Autodesk Fusion 360 part; units mm, degrees
sketch "Sketch3" plane through (0, 0, 0) normal (0, 0, 1) x (1, 0, 0)
  circle A0 centre (0, 0) radius 5.75
  dimension "d17" = 11.5
ref_plane "WorkPlane1" through (0, 0, 46) normal (0, 0, 1) x (1, 0, 0)
sketch "Sketch4" plane through (0, 0, 46) normal (0, 0, 1) x (1, 0, 0)
  line L0 (4, -6) -> (-4, -6)
  line L1 (-6, -4) -> (-6, 4)
  line L2 (-4, 6) -> (4, 6)
  line L3 (6, 4) -> (6, -4)
  arc A0 (-4, 6) -> (-6, 4) centre (-4, 4) ccw
  arc A1 (6, 4) -> (4, 6) centre (4, 4) ccw
  arc A2 (4, -6) -> (6, -4) centre (4, -4) ccw
  arc A3 (-6, -4) -> (-4, -6) centre (-4, -4) ccw
  point P0 (-6, -6)
  point P1 (-6, 6)
  point P2 (6, 6)
  dimension "d19" = 12
  dimension "d20" = 12
  dimension "d21" = 6
  dimension "d22" = 6
  dimension "d23" = 2
  dimension "d24" = 2
  dimension "d25" = 2
  dimension "d26" = 2
loft "Loft1" add profiles "Sketch3", "Sketch4" section 1 section 2
sketch "Sketch5" plane through (0, 0, 0) normal (0, 0, -1) x (1, 0, 0)
  circle A0 centre (0, 0) radius 4.75
  arc A1 (4.8644, 3.066) -> (4.8549, -3.081) centre (0, 0) ccw
  arc A2 (4.8549, -3.081) -> (4.8644, 3.066) centre (0, 0) ccw
  dimension "d27" = 9.5
extrude "Extrude2" cut sketch "Sketch5" against normal blind 43 contours A0
fillet "Fillet1" radius 1 2 edges at (6, 0, 46) (-6, 0, 46)
fillet "Fillet2" radius 0.5 1 edges at (-4.4286, -1.7177, 0)
sketch "Sketch1" plane through (0, 0, 0) normal (0, 1, 0) x (1, 0, 0)
  circle A0 centre (0, 0) radius 4.5
  circle A1 centre (0, 0) radius 5.5
  dimension "d1" = 9
  dimension "d2" = 11
extrude "Extrude1" [suppressed]
sketch "Sketch2" plane through (0, 0, 0) normal (0, 0, 1) x (1, 0, 0)
  line L0 (4.75, 0) -> (4.75, 43)
  line L1 (4.75, 43) -> (0, 43)
  line L2 (0, 43) -> (0, 45)
  line L3 (0, 45) -> (5.75, 45)
  line L4 (5.75, 45) -> (5.75, 0)
  line L5 (5.75, 0) -> (4.75, 0)
  dimension "d6" = 43
  dimension "d7" = 2
  dimension "d8" = 1
  dimension "d10" = 4.75
  dimension "d14" = 4.75
revolve "Revolve3" [suppressed]
chamfer "Chamfer1" [suppressed]
revolve "Revolve1" [suppressed]
revolve "Revolve2" [suppressed]
equation "d17 = ( ( ( 4.75 * 2 ) * 1 ) * 1 mm ) + 2 mm"
equation "d27 = ( 4.75 * 2 ) * 1 mm"
Work out the finished part from the listing and answer in its coordinate system (mm). Round coordinates to 2 decimals unless told otherwise and drop trailing zeros. Use one line per item in the form item = value. Start each with the question number.
(1) Flat-ended cylindrical pins translate along their axes: P1, Ø2, axis at y = 2, z = 5.5, coming from the -X side; P2, Ø5, axis at y = 2, z = 21.5, coming from the +X side; P3, Ø5, axis at y = -2, z = 6.5, coming from the +X side. Find the tip coordinate at first contact, or state that the pin passes through.
(2) Consider line 1 (Z direction, x = -3.25, y = 2.5); line 2 (Y direction, x = 0, z = 28); line 3 (X direction, y = -3.25, z = 18). Determine where each line is inside the solid, lowest interval first.
(3) Determine the mould class of faces 1 (the face through (0, 0, 43)), 2 (the face through (0, 0, 46)) for opening direction X: +X half, -X half, draft (parallel to the pull), parting line (faces both ways), or undercut.
Answer list:
q1.P1 = -5.71
q1.P2 = 5.88
q1.P3 = 5.79
q2.line_1 = 43 to 46
q2.line_2 = -5.9 to -4.75, 4.75 to 5.9
q2.line_3 = -5.35 to -3.46, 3.46 to 5.35
q3.face_1 = undercut
q3.face_2 = draft
